Here's how the part is built. I have some questions about the finished solid (model axes, mm). Face numbers are marked on the shaded views. Round coordinates to 2 decimals unless told otherwise and drop trailing zeros. Write each loop counter-clockwise with the first axis right and the second up, starting at its lowest first coordinate (ties: lowest second). Pieces come first, ordered by that corner, then holes. Notation, with made-up numbers: (-14, -35) - (-6, -35) arc R16 cw to (-6, -28) - close; hole circle Ø10 at (82, -29.75). An arc over 180 degrees is marked (long way). One line per item, written item: value. Start each with the question number.
Item 1: If I drill on line 1 (Y direction, x = 46, z = 4.5); line 2 (X direction, y = 52, z = 3); line 3 (Y direction, x = 23.5, z = 6), over which ranges is the centre line in solid material (lowest first)?
Item 2: Imagine slicing it at C-C, the plane x = 16. Please give me the cut outline in (y, z), then the cut area to 3 significant figures.
Item 3: Imagine slicing it at B-B, the plane y = 34.5. Please give me the cut outline in (x, z).
Item 4: For P1, Ø0.6, axis at x = 47.5, y = 1, coming from the +Z side; P2, Ø1.2, axis at y = 0.5, z = 7, coming from the -X side; P3, Ø1.1, axis at y = 1, z = 7.5, coming from the +X side, each with a flat end and sliding along its axis, tell me the tip position at first contact or that it passes through.
Item 5: Thinking about a two-plate mould opening in X: for the marked faces 1 and 2, which applies, released by +X, released by -X, zero draft, split by the parting line, or undercut?
Item 6: Imagine slicing it at A-A, the plane z = 3.75. Please give me the cut outline in (x, y).
```python
from build123d import *

# Parameters (mm, degrees)
BOX_W           = 59
BOX_H           = 90
BOX_DEPTH       = 8
SKETCH_W        = 55
SKETCH_H        = 86
POCKET_DEPTH    = 6
POCKET001_DEPTH = 2
FILLET_R        = 2
FILLET002_R     = 2


with BuildPart() as part:
    # Box → Box (join)
    with BuildSketch(Plane.XY):
        with Locations((29.5, 45)):
            Rectangle(BOX_W, BOX_H)
    extrude(amount=BOX_DEPTH)

    # Sketch (on Face6 of Box) → Pocket (cut)
    with BuildSketch(Plane.XY.offset(8)):
        with Locations((29.5, 45)):
            Rectangle(SKETCH_W, SKETCH_H)
    extrude(amount=-POCKET_DEPTH, mode=Mode.SUBTRACT)

    # Sketch001 (on Face2 of Pocket) → Pocket001 (cut)
    with BuildSketch(Plane.XZ):
        with BuildLine():
            Line((28.5, 8), (28.5, 7))
            ThreePointArc((26.5, 5), (27.914214, 5.585786), (28.5, 7))
            Line((26.5, 5), (21.5, 5))
            ThreePointArc((19.5, 7), (20.085786, 5.585786), (21.5, 5))
            Line((19.5, 7), (19.5, 8))
            Line((19.5, 8), (28.5, 8))
        make_face()
        with BuildLine():
            ThreePointArc((45, 6.5), (45.43934, 5.43934), (46.5, 5))
            Line((46.5, 5), (49.5, 5))
            ThreePointArc((49.5, 5), (50.56066, 5.43934), (51, 6.5))
            Line((51, 6.5), (51, 8))
            Line((45, 8), (51, 8))
            Line((45, 6.5), (45, 8))
        make_face()
    extrude(amount=-POCKET001_DEPTH, mode=Mode.SUBTRACT)

    # Fillet
    fillet_edges = [part.edges().sort_by_distance(p)[0] for p in [
        (59, 90, 4),
        (0, 90, 4),
        (0, 0, 4),
        (59, 0, 4),
    ]]
    fillet(fillet_edges, radius=FILLET_R)

    # Fillet002
    fillet002_edges = [part.edges().sort_by_distance(p)[0] for p in [
        (29.5, 0, 0),
    ]]
    fillet(fillet002_edges, radius=FILLET002_R)


solid = part.part
```
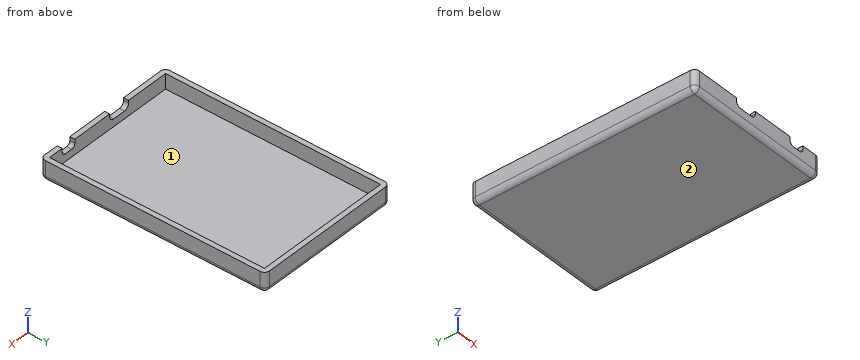
Values follow:
1. line 1: y = 0 to 2, 88 to 90
1. line 2: x = 0 to 2, 57 to 59
1. line 3: y = 88 to 90
2. outline: (0, 2) arc R2 ccw to (2, 0) - (88, 0) arc R2 ccw to (90, 2) - (90, 8) - (88, 8) - (88, 2) - (2, 2) - (2, 8) - (0, 8) - close
2. area: 202 mm^2
3. outline: (0, 2) arc R2 ccw to (2, 0) - (57, 0) arc R2 ccw to (59, 2) - (59, 8) - (57, 8) - (57, 2) - (2, 2) - (2, 8) - (0, 8) - close
4. P1: stops at z = 5
4. P2: stops at x = 0.21
4. P3: stops at x = 58.95
5. face 1: undercut
5. face 2: zero draft
6. outline: (0, 2) arc R2 ccw to (2, 0) - (57, 0) arc R2 ccw to (59, 2) - (59, 88) arc R2 ccw to (57, 90) - (2, 90) arc R2 ccw to (0, 88) - close; hole (2, 2) - (57, 2) - (57, 88) - (2, 88) - close
